Read the model definition and answer for the solid it produces. Units are mm, in the model's axes. Face numbers are marked on the shaded views. Give positions to 0.01 mm unless a question says otherwise; leave off trailing zeros. Order: outer loops, then holes, each group sorted by start corner. A loop starts at its lowest first (then second) coordinate and runs counter-clockwise, first axis right, second up. Notation, with made-up numbers: (2, 35.25) - (49, 35.25) arc R19 ccw to (49, 51.25) - close; hole circle Ø8 at (50, 60.5). An arc over 180 degrees is marked (long way). Write each question's results on one line, items separated by ' | '.
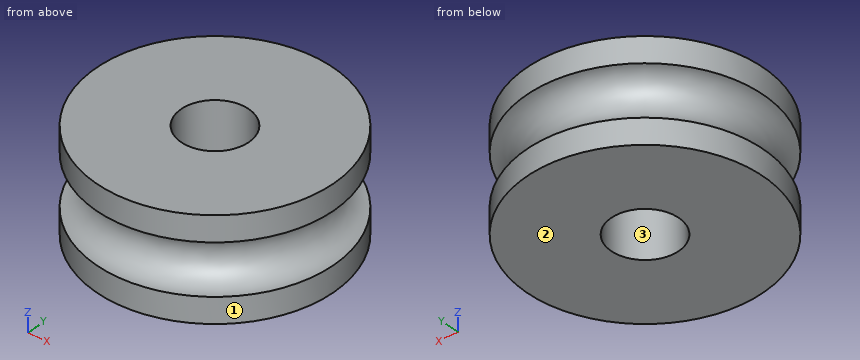
from build123d import *

# Parameters (mm, degrees)
CROQUIS1_R              = 3.5
SALIENTE_EXTRUIR1_DEPTH = 3
CROQUIS2_R              = 0.75
CROQUIS3_R              = 1
CORTAR_EXTRUIR1_DEPTH   = 6.787918451


with BuildPart() as part:
    # Croquis1 → Saliente-Extruir1 (new body)
    with BuildSketch(Plane.XY):
        Circle(CROQUIS1_R)
    extrude(amount=SALIENTE_EXTRUIR1_DEPTH)

    # Croquis2 → Cortar-Revolución1 (revolve, cut)
    with BuildSketch(Plane(origin=(0, 0, 0), x_dir=(0, 0, -1), z_dir=(1, 0, 0)), mode=Mode.PRIVATE) as cortar_revoluci_n1_sk:
        with Locations((-1.5, 3.5)):
            Circle(CROQUIS2_R)
    revolve(cortar_revoluci_n1_sk.sketch.rotate(Axis((0, 0, 3), (0, 0, -1)), 90), axis=Axis((0, 0, 3), (0, 0, -1)), mode=Mode.SUBTRACT)

    # Croquis3 → Cortar-Extruir1 (cut, through all)
    with BuildSketch(Plane.XY.offset(3)):
        Circle(CROQUIS3_R)
    extrude(amount=-CORTAR_EXTRUIR1_DEPTH, mode=Mode.SUBTRACT)


solid = part.part
(1) The mould has two halves that part along Y. Classify the marked faces 1, 2 and 3: pulls with the +Y half, pulls with the -Y half, needs draft (parallel to the pull), parting line crosses it, or undercut.
Conclusion:
face 1: parting line crosses it | face 2: needs draft | face 3: undercut
(2) Section A-A (x = 0) is taken. Give the vertices of the cut face in (y, z).
Conclusion:
outline: (-3.5, 0) - (-1, 0) - (-1, 3) - (-3.5, 3) - (-3.5, 2.25) arc R0.75 cw to (-3.5, 0.75) - close; (1, 0) - (3.5, 0) - (3.5, 0.75) arc R0.75 cw to (3.5, 2.25) - (3.5, 3) - (1, 3) - close
(3) Section C-C (z = 2.35) is taken. Give the vertices of the cut face in (x, y).
Conclusion:
outline: circle Ø7 at (0, 0); hole circle Ø2 at (0, 0)
(4) This flat-tipped pin is pushed along its axis until it touches: pin 1 (1.5 mm diameter, centred on x = 2.5, z = 2, fed in from +Y). Where does it stop, or does it pass through?
Conclusion:
pin 1: y = 3.01
(5) Consider probe 1 along Y at (x, z) = (0, 2.3); probe 2 along Y at (x, z) = (0.25, 1.55); probe 3 along Z at (x, y) = (1, -2.75). Determine where each line is inside the solid, lowest interval first. Write a range as [from, to].
Conclusion:
probe 1: [-3.5, -1], [1, 3.5] | probe 2: [-2.74, -0.97], [0.97, 2.74] | probe 3: [0, 1.02], [1.98, 3]
(6) Section D-D (z = 1.7) is taken. Give the vertices of the cut face in (x, y), plus the area to 3 significant figures.
Conclusion:
outline: circle Ø5.55 at (0, 0); hole circle Ø2 at (0, 0) | area: 21.1 mm^2
